The model under review builds one solid part; all positions refer to its coordinate system, in mm. A direction names the side the tool comes from. Round coordinates to 2 decimals unless told otherwise and drop trailing zeros. Order: outer loops, then holes, each group sorted by start corner. A loop starts at its lowest first (then second) coordinate and runs counter-clockwise, first axis right, second up.
1) Clearance check with flat-ended pins moving along their axes: P1, Ø1.5, axis at x = 248, z = -63.5, coming from the +Y side; P2, Ø1, axis at x = 156.5, z = 2.5, coming from the +Y side; P3, Ø1.6, axis at x = 16.5, z = 1, coming from the +Y side; P4, Ø1.6, axis at x = 157, z = 2, coming from the -Y side. State where each tip first meets the part, or that it passes through.
2) Machinability: for faces 5 (the face through (153, 82, 3.175)), 6 (the face through (153, 82, 0)), which of the approach directions +Z, -Z, +X, -X, +Y, -Y give a long, thin tool a straight path to every point of the face, cutting with its end or side? Answer none if there is none.
3) Consider section D-D (y = 206). Give the boundary of the cut face in (x, z) (3 decimals), then the cut area to 3 significant figures.
4) Consider section A-A (y = 25.4). Give the boundary of the cut face in (x, z) (3 decimals).
5) To check wall thickness, follow L1, parallel to Y at x = 44.45, z = 1.05; L2, parallel to Z at x = 71, y = 46 (3 decimals); L3, parallel to Z at x = 145.5, y = 187. State the ranges of each line that lie inside material, in increasing order.
6) Consider section C-C (z = -9). Give the boundary of the cut face in (x, y) (3 decimals).
7) Consider section B-B (x = 145.5). Give the boundary of the cut face in (y, z) (3 decimals).
8) Mouldability with a two-part tool opening along Y and no side actions: class faces 1 (the face through (174.48, 146.174, 1.565)), 2 (the face through (34.54, 208.56, -51.12)), 3 (the face through (157.8, 195.83, -38.39)), 4 (the face through (55, 29.8, 1.6)) as pulls with the +Y half, pulls with the -Y half, needs draft (parallel to the pull), parting line crosses it, or undercut.
Autodesk Inventor part; units mm, degrees
ref_plane "YZ Plane" through (0, 0, 0) normal (1, 0, 0) x (0, 1, 0)
ref_plane "XZ Plane" through (0, 0, 0) normal (0, 1, 0) x (-1, 0, 0)
ref_plane "XY Plane" through (0, 0, 0) normal (0, 0, 1) x (1, 0, 0)
sketch "Sketch1" plane through (0, 0, 0) normal (0, 0, 1) x (1, 0, 0)
  arc A0 (-3.175, 3.175) -> (0, 0) centre (0, 3.175) ccw
  line L0 (0, 0) -> (311.15, 0)
  arc A1 (311.15, 0) -> (314.325, 3.175) centre (311.15, 3.175) ccw
  line L1 (314.325, 3.175) -> (314.325, 161.925)
  line L2 (311.15, 165.1) -> (12.1553, 165.1)
  line L3 (-3.175, 149.7697) -> (-3.175, 3.175)
  line L4 (292.1, 12.065) -> (298.45, 12.065)
  arc A2 (298.45, 6.985) -> (298.45, 12.065) centre (298.45, 9.525) ccw
  line L5 (298.45, 6.985) -> (292.1, 6.985)
  arc A3 (292.1, 12.065) -> (292.1, 6.985) centre (292.1, 9.525) ccw
  line L6 (302.26, 47.625) -> (302.26, 53.975)
  arc A4 (307.34, 53.975) -> (302.26, 53.975) centre (304.8, 53.975) ccw
  line L7 (307.34, 53.975) -> (307.34, 47.625)
  arc A5 (302.26, 47.625) -> (307.34, 47.625) centre (304.8, 47.625) ccw
  line L8 (152.4, 12.065) -> (158.75, 12.065)
  arc A6 (158.75, 6.985) -> (158.75, 12.065) centre (158.75, 9.525) ccw
  line L9 (158.75, 6.985) -> (152.4, 6.985)
  arc A7 (152.4, 12.065) -> (152.4, 6.985) centre (152.4, 9.525) ccw
  line L10 (12.7, 12.065) -> (19.05, 12.065)
  arc A8 (19.05, 6.985) -> (19.05, 12.065) centre (19.05, 9.525) ccw
  line L11 (19.05, 6.985) -> (12.7, 6.985)
  arc A9 (12.7, 12.065) -> (12.7, 6.985) centre (12.7, 9.525) ccw
  line L12 (302.26, 142.875) -> (302.26, 149.225)
  arc A10 (307.34, 149.225) -> (302.26, 149.225) centre (304.8, 149.225) ccw
  line L13 (307.34, 149.225) -> (307.34, 142.875)
  arc A11 (302.26, 142.875) -> (307.34, 142.875) centre (304.8, 142.875) ccw
  line L14 (0.2503, 82.1064) -> (1.9189, 86.7699)
  arc A12 (6.4628, 85.1441) -> (1.9189, 86.7699) centre (4.1909, 85.957) ccw
  line L15 (6.4628, 85.1441) -> (4.7942, 80.4806)
  arc A13 (0.2503, 82.1064) -> (4.7942, 80.4806) centre (2.5223, 81.2935) ccw
  line L16 (28.2458, 146.0235) -> (26.5772, 141.36)
  arc A14 (22.0333, 142.9859) -> (26.5772, 141.36) centre (24.3053, 142.1729) ccw
  line L17 (22.0333, 142.9859) -> (23.702, 147.6493)
  arc A15 (28.2458, 146.0235) -> (23.702, 147.6493) centre (25.9739, 146.8364) ccw
  circle A16 centre (88.302, 150.3688) radius 2.5797
  circle A17 centre (66.077, 140.8438) radius 2.5797
  circle A18 centre (43.852, 150.3688) radius 2.5797
  circle A19 centre (273.2565, 61.6719) radius 2.413
  circle A20 centre (252.6531, 41.0685) radius 2.413
  circle A21 centre (277.6672, 36.6578) radius 2.413
  circle A22 centre (44.45, 25.4) radius 11.43
  line L18 (12.1553, 165.1) -> (-3.175, 165.1)
  line L19 (-3.175, 165.1) -> (-3.175, 149.7697)
  line L20 (314.325, 161.925) -> (314.325, 165.1)
  line L21 (314.325, 165.1) -> (311.15, 165.1)
  point P0 (0, 0)
  point P1 (-3.175, 3.175)
  point P2 (0, 0)
  point P3 (314.325, 3.175)
  point P4 (22.0333, 142.9859)
  point P5 (23.702, 147.6493)
  point P6 (28.2458, 146.0235)
  point P7 (26.5772, 141.36)
  point P8 (6.4628, 85.1441)
  point P9 (19.05, 6.985)
  point P10 (158.75, 6.985)
  point P11 (298.45, 6.985)
  dimension "GapSize" = 3.175
extrude "Plate1" add sketch "Sketch1" along normal blind 3.175
sketch "Sketch2" plane through (314.325, 162.6678, 1.1341) normal (0, 0.7660444, 0.6427876) x (-1, 0, 0)
  line L0 (317.5, 0) -> (0, 0)
  line L1 (0, 0) -> (0, -101.6)
  line L2 (0, -101.6) -> (317.5, -101.6)
  line L3 (317.5, -101.6) -> (317.5, 0)
edge flange "Flange1" height 101.6 angle 50 thickness 3.175 bend radius 3.175 thickness toward (0, 0.7660444, 0.6427876) relief tear relief width 3.175 relief depth 1.5875 edges at (161.6526, 165.1, 0) wall of the first edge with corners at (-3.175, 162.6678, 1.1341) (314.325, 162.6678, 1.1341) (314.325, 227.975, -76.696) (-3.175, 227.975, -76.696)
bend "Bend1"
corner "Corner1"
chamfer "Corner Chamfer1" distance 76.2 distance2 63.5 1 edges at (-3.175, 229.1911, -75.6755) measured on face at (102.6583, 228.7858, -76.0157)
sketch "Sketch3" plane through (0, 0, 3.175) normal (0, 0, 1) x (1, 0, 0)
  line L0 (311.15, 0) -> (0, 0)
  line L1 (-3.175, 3.175) -> (-3.175, 162.1389)
  point P0 (174.625, 142.875)
  dimension "d149" = 142.875
  dimension "d150" = 177.8
hole "Hole1" at (174.625, 142.875, 3.175) direction (0, 0, -1) diameter 6.604 end through all
fillet "Corner Round1" radius 3.175 3 edges at (314.325, 229.1911, -75.6755) (73.025, 229.1911, -75.6755) (-3.175, 188.3741, -27.0317)
equation "\"GapSize\" = Thickness"
equation "\"d156\" = Thickness"
equation "\"d135\" = Thickness"
equation "\"d136\" = BendReliefWidth"
equation "\"d137\" = BendReliefDepth"
equation "\"d138\" = MinimumRemnant"
equation "\"d139\" = TransitionRadius"
equation "\"d142\" = BendRadius"
equation "\"d143\" = CornerReliefSize"
equation "\"d144\" = GapSize"
equation "\"d145\" = JacobiRadiusSize"
equation "\"BendRadius\" = Thickness"
equation "\"BendReliefWidth\" = Thickness"
equation "\"BendReliefDepth\" = 0.5 * Thickness"
equation "\"CornerReliefSize\" = 4 * Thickness"
equation "\"MinimumRemnant\" = 2 * Thickness"
equation "\"TransitionRadius\" = BendRadius"
equation "\"JacobiRadiusSize\" = BendRadius"
properties part number "TURRET,WIRE,PLATE,BOTTOM" material "Polycarbonate, Clear"
Answer below:
1. P1: stops at y = 221.68
1. P2: stops at y = 165.82
1. P3: stops at y = 167.6
1. P4: stops at y = 0
2. face 5: +Z, +X, -X, +Y, -Y
2. face 6: -Z, +X, -X, -Y
3. outline: (27.46, -45.568) - (32.001, -50.507) - (314.325, -50.507) - (314.325, -45.568) - close
3. area: 1,410 mm2
4. outline: (-3.175, 0) - (33.02, 0) - (33.02, 3.175) - (-3.175, 3.175) - close; (55.88, 0) - (314.325, 0) - (314.325, 3.175) - (55.88, 3.175) - close
5. L1: y = 0 to 13.97, 36.83 to 147.86, 152.88 to 166.88
5. L2: z = 0 to 3.175
5. L3: z = -27.86 to -22.92
6. outline: (-3.175, 171.171) - (314.325, 171.171) - (314.325, 175.316) - (-3.175, 175.316) - close
7. outline: (0, 0) - (162.139, 0) arc R3.175 cw to (164.571, -1.134) - (227.975, -76.696) - (230.407, -74.655) - (167.003, 0.907) arc R6.35 ccw to (162.139, 3.175) - (0, 3.175) - close
8. face 1: undercut
8. face 2: pulls with the +Y half
8. face 3: pulls with the -Y half
8. face 4: undercut
